from build123d import *

# Parameters (mm, degrees)
SKETCH1_W           = 25.4
SKETCH1_H           = 10.16
BOSS_EXTRUDE1_DEPTH = 101.6
SKETCH2_R           = 6.35
CUT_EXTRUDE1_DEPTH  = 88.9
SKETCH5_W           = 12.7
SKETCH5_H           = 28.575
CUT_EXTRUDE3_DEPTH  = 15.875
FILLET1_R           = 6.35


with BuildPart() as part:
    # Sketch1 → Boss-Extrude1 (new body)
    with BuildSketch(Plane.XY):
        with Locations((0, 5.08)):
            Rectangle(SKETCH1_W, SKETCH1_H)
    extrude(amount=BOSS_EXTRUDE1_DEPTH)

    # Sketch2 → Cut-Extrude1 (cut)
    with BuildSketch(Plane(origin=(0, 10.16, 0), x_dir=(1, 0, 0), z_dir=(0, 1, 0))):
        with Locations(Location((0, -50.8, 0), (0, 0, 180))):
            Circle(SKETCH2_R)
    extrude(amount=-CUT_EXTRUDE1_DEPTH, mode=Mode.SUBTRACT)

    # Sketch5 → Cut-Extrude3 (cut)
    with BuildSketch(Plane(origin=(0, 10.16, 0), x_dir=(1, 0, 0), z_dir=(0, 1, 0))):
        with Locations((0, -77.7875)):
            Rectangle(SKETCH5_W, SKETCH5_H)
        with Locations((0, -23.8125)):
            Rectangle(SKETCH5_W, SKETCH5_H)
    extrude(amount=-CUT_EXTRUDE3_DEPTH, mode=Mode.SUBTRACT)

    # Fillet1
    fillet1_edges = [part.edges().sort_by_distance(p)[0] for p in [
        (-6.35, 5.08, 92.075),
        (-6.35, 5.08, 38.1),
        (-6.35, 5.08, 63.5),
        (-6.35, 5.08, 9.525),
        (6.35, 5.08, 9.525),
        (6.35, 5.08, 63.5),
        (6.35, 5.08, 92.075),
        (6.35, 5.08, 38.1),
    ]]
    fillet(fillet1_edges, radius=FILLET1_R - 0.0001)  # a hair under: the kernel refuses the full size


solid = part.part
Check sheet for the modelled part. Datum: model origin and axes. Units: mm. A direction names the side the tool comes from. Give positions to 0.01 mm unless a question says otherwise; leave off trailing zeros. Write each loop counter-clockwise with the first axis right and the second up, starting at its lowest first coordinate (ties: lowest second). Pieces come first, ordered by that corner, then holes. Notation, with made-up numbers: M -15,25.5 L 24,25.5 A20 ccw 24,41.5 Z; hole C 87.25,11 d6. An arc over 180 degrees is marked long. Use one line per item in the form item = value.
(1) Section check A-A on y = 6.75. State how many separate pieces and enclosed holes the cut face has, plus the area to 3 significant figures.
Answer block:
separate_pieces = 1
enclosed_holes = 3
area = 1,800 mm2
(2) Draft check along X on faces 1 (the flat face through (-12.7, 5, 50)), 2 (the flat face through (12.7, 5, 50)), 3 (the cylindrical face through (4.44, 5.01, 36.29)). Enter one of: pulls with the +X half, pulls with the -X half, needs draft (parallel to the pull), parting line crosses it, or undercut.
Answer block:
face_1 = pulls with the -X half
face_2 = pulls with the +X half
face_3 = undercut
(3) Section check C-C on x = 2.5. Record the boundary of the cut face in (y, z).
Answer block:
outline = M 0,0 L 10.16,0 L 10.16,10.04 L 0,10.04 Z; M 0,37.59 L 10.16,37.59 L 10.16,44.96 L 0,44.96 Z; M 0,56.64 L 10.16,56.64 L 10.16,64.01 L 0,64.01 Z; M 0,91.56 L 10.16,91.56 L 10.16,101.6 L 0,101.6 Z
(4) Section check B-B on z = 50.8. Record the boundary of the cut face in (x, y), plus the area to 3 significant figures.
Answer block:
outline = M -12.7,0 L -6.35,0 L -6.35,10.16 L -12.7,10.16 Z; M 6.35,0 L 12.7,0 L 12.7,10.16 L 6.35,10.16 Z
area = 129 mm2
(5) Depth check by flat-ended pin: P1, Ø8, axis at x = 0.5, z = 25.5, coming from the +Y side. Enter the tip coordinate at first touch or a pass-through.
Answer block:
P1 = through
(6) Tool access check on faces 4 (the flat face through (8, 0, 50)), 5 (the flat face through (-6.35, 5, 24)). Record the directions out of +Z, -Z, +X, -X, +Y, -Y that give a thin tool (end or side, any length) a straight path to the whole face; none if there is none.
Answer block:
face_4 = +Z, -Z, +X, -X, -Y
face_5 = +Y, -Y
(7) Material ranges on line 1 along Z through (x, y) = (0, 5) (3 decimals); line 2 along Z through (x, y) = (-4, 0.5); line 3 along X through (y, z) = (2.75, 82.5), recorded low to high.
Answer block:
line_1 = 0 to 9.525, 38.1 to 44.45, 57.15 to 63.5, 92.075 to 101.6
line_2 = 0 to 10.94, 36.68 to 45.87, 55.73 to 64.92, 90.66 to 101.6
line_3 = -12.7 to -6.35, 6.35 to 12.7
